```python
from build123d import *

# Parameters (mm, degrees)
F1_DEPTH = 6.35
F3_DEPTH = 76.2
F4_R     = 20.270686
F5_DEPTH = 104.346251
F6_R     = 3.175
F7_DEPTH = 180.547251


with BuildPart() as f1:
    # F0 (on Top) → F1 (new body)
    with BuildSketch(Plane.XY):
        Polygon((-82.839586, 50.360938), (-82.839586, 0), (82.839586, 0), (82.839586, 50.360938), (54.840428, 76.2), (-54.840428, 76.2), align=None)
    extrude(amount=F1_DEPTH)

    # F2 (on face) → F3 (join)
    with BuildSketch(Plane(origin=(0, 0, 0), x_dir=(1, 0, 0), z_dir=(0, 0, -1))):
        Polygon((-54.840428, -76.2), (54.840428, -76.2), (82.839586, -50.360938), (79.094327, -50.360938), (53.847508, -73.66), (-53.847508, -73.66), (-79.094327, -50.360938), (-82.839586, -50.360938), align=None)
    extrude(amount=F3_DEPTH)

    # F4 (on face) → F5 (join)
    with BuildSketch(Plane(origin=(0, 0, 0), x_dir=(1, 0, 0), z_dir=(0, 0, -1))):
        with Locations((-6.616414, -35.295554)):
            Circle(F4_R)
    extrude(amount=-F5_DEPTH)

    # F6 (on face) → F7 (cut, through all)
    with BuildSketch(Plane.XY.offset(104.346251)):
        with Locations((0, 38.975005)):
            Circle(F6_R)
    extrude(amount=-F7_DEPTH, mode=Mode.SUBTRACT)


solid = f1.part
```
The listing builds one solid part. Answer for the finished solid, in the listing's coordinates (mm). A direction names the side the tool comes from. Give positions to 0.01 mm unless a question says otherwise; leave off trailing zeros. Order: outer loops, then holes, each group sorted by start corner. A loop starts at its lowest first (then second) coordinate and runs counter-clockwise, first axis right, second up. Notation, with made-up numbers: (-40, -34.75) -> (17, -34.75) arc R7 ccw to (17, -22.75) -> close; hole circle Ø10 at (45.25, 35). An arc over 180 degrees is marked (long way). Write each question's results on one line, items separated by ' | '.
Q1. Straight lines are drawn through the part: probe 1 along Z at (x, y) = (9.5, 24); probe 2 along Z at (x, y) = (8.5, 57); probe 3 along X at (y, z) = (72, -13.5). For each, find the intervals that lie inside material, in ascending order. Write a range as from..to.
Checked values:
probe 1: z = 0..104.35 | probe 2: z = 0..6.35 | probe 3: x = -59.39..-55.65, 55.65..59.39
Q2. The part is cut by section A-A, the plane z = -62. Give the vertices of the cut face in (x, y), and give its area (3 significant figures).
Checked values:
outline: (-82.84, 50.36) -> (-79.09, 50.36) -> (-53.85, 73.66) -> (53.85, 73.66) -> (79.09, 50.36) -> (82.84, 50.36) -> (54.84, 76.2) -> (-54.84, 76.2) -> close | area: 460 mm^2
Q3. The part is cut by section B-B, the plane x = 0. Give the vertices of the cut face in (y, z).
Checked values:
outline: (0, 0) -> (35.8, 0) -> (35.8, 104.35) -> (16.14, 104.35) -> (16.14, 6.35) -> (0, 6.35) -> close; (42.15, 0) -> (73.66, 0) -> (73.66, -76.2) -> (76.2, -76.2) -> (76.2, 6.35) -> (54.46, 6.35) -> (54.46, 104.35) -> (42.15, 104.35) -> close
Q4. Each of these flat-tipped pins is pushed along its axis until it touches: P1, Ø4, axis at y = 51, z = 18.5, coming from the +X side; P2, Ø10, axis at y = 50, z = 83, coming from the +X side; P3, Ø4, axis at x = 81.5, z = -49.5, coming from the -Y side; P4, Ø5.5, axis at x = 0, y = 38.98, coming from the +Z side. Where does it stop, or does it pass through?
Checked values:
P1: stops at x = 8.32 | P2: stops at x = 11.18 | P3: stops at y = 50.36 | P4: passes through
Q5. The part is cut by section C-C, the plane y = 58. Give the vertices of the cut face in (x, z).
Checked values:
outline: (-74.56, -76.2) -> (-70.82, -76.2) -> (-70.82, 0) -> (70.82, 0) -> (70.82, -76.2) -> (74.56, -76.2) -> (74.56, 6.35) -> (-74.56, 6.35) -> close
Q6. Determine the mould class of faces 1 (the face through (1, 73.66, -38)), 2 (the face through (-7, 35, 104.346)), 3 (the face through (68.6, 63.5, -34.3)), 4 (the face through (-66.294, 62.174, -37.567)) for opening direction X: pulls with the +X half, pulls with the -X half, needs draft (parallel to the pull), parting line crosses it, or undercut.
Checked values:
face 1: undercut | face 2: needs draft | face 3: pulls with the +X half | face 4: undercut
Q7. The part is cut by section D-D, the plane x = 32. Give the vertices of the cut face in (y, z).
Checked values:
outline: (0, 0) -> (73.66, 0) -> (73.66, -76.2) -> (76.2, -76.2) -> (76.2, 6.35) -> (0, 6.35) -> close
Q8. Which of the six approach directions +Z, -Z, +X, -X, +Y, -Y give full straight-line access (tool end or side, diameter ignored) to faces 5 (the face through (-11.011, 55.084, 54.662)), 6 (the face through (66.648, 61.847, -37.567)), 7 (the face through (82.84, 25, 3))?
Checked values:
face 5: +Z | face 6: -Z, -Y | face 7: +Z, -Z, +X, +Y, -Y
